CAD build for the part. Positions are in the model's coordinates, mm. Coordinates: 2 decimals unless noted, no trailing zeros. Write each loop counter-clockwise with the first axis right and the second up, starting at its lowest first coordinate (ties: lowest second). Pieces come first, ordered by that corner, then holes. Notation, with made-up numbers: (-31.5, -2) -> (-12.5, -2) arc R18 ccw to (-12.5, 23) -> close; hole circle Ø2 at (66, 7.5). An arc over 180 degrees is marked (long way). Answer as CSV lines item,"result".
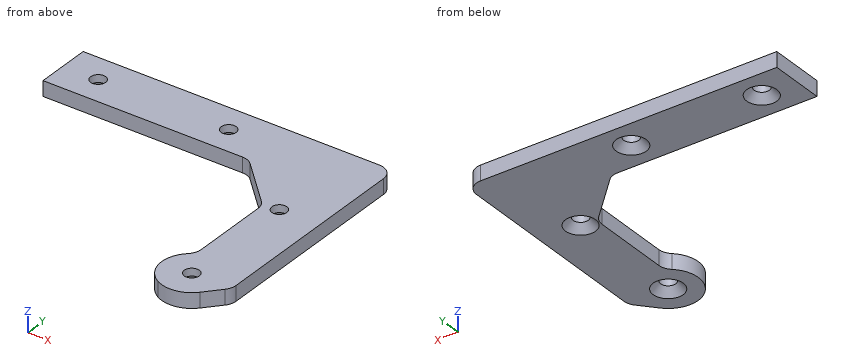
```python
from build123d import *

# Parameters (mm, degrees)
EXTRUDE_598_DEPTH      = 3
SKETCH_656_R           = 1.5
CUT_EXTRUDE_1014_DEPTH = 74.235920149
SKETCH_3_R             = 6
SKETCH_3_R_2           = 1.5
EXTRUDE_1306_DEPTH     = 3
CUT_EXTRUDE_1628_DEPTH = 74.235920149
CHAMFER_3_SIZE         = 10
FILLET_3_R             = 3
CHAMFER_2_SIZE         = 1.5


with BuildPart() as part:
    # Эскиз1 → Extrude 598 (new body)
    with BuildSketch(Plane.XY):
        Polygon((-56.5, 5.5), (-56.5, -5.5), (-5.5, -5.5), (-5.5, -46.5), (5.5, -46.5), (5.5, 5.5), align=None)
    extrude(amount=EXTRUDE_598_DEPTH)

    # Sketch 656 → Cut-Extrude 1014 (cut, through all)
    with BuildSketch(Plane.XY.offset(3)):
        with Locations((-49.5, 0)):
            Circle(SKETCH_656_R)
        with Locations((-23.5, 0)):
            Circle(SKETCH_656_R)
        with Locations((-2.5, -15)):
            Circle(SKETCH_656_R)
        with Locations((-2.5, -39)):
            Circle(SKETCH_656_R)
    extrude(amount=-CUT_EXTRUDE_1014_DEPTH, mode=Mode.SUBTRACT)

    # Эскиз3 → Extrude 1306 (add)
    with BuildSketch(Plane.XY.offset(3)):
        with Locations((-2.5, -39)):
            Circle(SKETCH_3_R)
        with Locations((-2.5, -39)):
            Circle(SKETCH_3_R_2, mode=Mode.SUBTRACT)
    extrude(amount=-EXTRUDE_1306_DEPTH)

    # Эскиз4 → Cut-Extrude 1628 (cut, through all)
    with BuildSketch(Plane.XY.offset(3)):
        with BuildLine():
            Line((-5.5, -46.5), (-5.5, -44.196152423))
            ThreePointArc((-5.5, -44.196152423), (-1.530874267, -44.921215696), (2, -42.968626967))
            Line((2, -42.968626967), (5.5, -39))
            Line((5.5, -39), (5.5, -46.5))
            Line((5.5, -46.5), (-5.5, -46.5))
        make_face()
    extrude(amount=-CUT_EXTRUDE_1628_DEPTH, mode=Mode.SUBTRACT)

    # Фаска3
    chamfer_3_edges = [part.edges().sort_by_distance(p)[0] for p in [
        (-5.5, -5.5, 1.5),
    ]]
    chamfer(chamfer_3_edges, length=CHAMFER_3_SIZE)

    # Скругление3
    fillet_3_edges = [part.edges().sort_by_distance(p)[0] for p in [
        (5.5, 5.5, 1.5),
        (-5.5, -33.803847577, 1.5),
        (5.5, -39, 1.5),
        (-5.5, -15.5, 1.5),
        (-15.5, -5.5, 1.5),
    ]]
    fillet(fillet_3_edges, radius=FILLET_3_R)

    # Фаска2
    chamfer_2_edges = [part.edges().sort_by_distance(p)[0] for p in [
        (-4, -15, 0),
        (-51, 0, 0),
        (-25, 0, 0),
        (-4, -39, 0),
    ]]
    chamfer(chamfer_2_edges, length=CHAMFER_2_SIZE)


solid = part.part
```
Item 1: Saw through at A-A on x = -2.5. Give the cut face in (y, z), and give its area (3 significant figures).
Answer below:
outline,"(-45, 0) -> (-42, 0) -> (-40.5, 1.5) -> (-40.5, 3) -> (-45, 3) -> close; (-37.5, 1.5) -> (-36, 0) -> (-18, 0) -> (-16.5, 1.5) -> (-16.5, 3) -> (-37.5, 3) -> close; (-13.5, 1.5) -> (-12, 0) -> (5.5, 0) -> (5.5, 3) -> (-13.5, 3) -> close"
area,"129 mm2"
Item 2: Saw through at C-C on z = 0.95. Give the cut face in (x, y).
Answer below:
outline,"(-56.5, -5.5) -> (-16.74, -5.5) arc R3 cw to (-14.62, -6.38) -> (-6.38, -14.62) arc R3 cw to (-5.5, -16.74) -> (-5.5, -32.29) arc R3 cw to (-6.5, -34.53) arc R6 ccw (long way) to (2, -42.97) -> (4.75, -39.85) arc R3 ccw to (5.5, -37.87) -> (5.5, 2.5) arc R3 ccw to (2.5, 5.5) -> (-56.5, 5.5) -> close; hole circle Ø4.1 at (-49.5, 0); hole circle Ø4.1 at (-23.5, 0); hole circle Ø4.1 at (-2.5, -39); hole circle Ø4.1 at (-2.5, -15)"
Item 3: Saw through at D-D on x = -23.5. Give the cut face in (y, z), and give its area (4 significant figures).
Answer below:
outline,"(-5.5, 0) -> (-3, 0) -> (-1.5, 1.5) -> (-1.5, 3) -> (-5.5, 3) -> close; (1.5, 1.5) -> (3, 0) -> (5.5, 0) -> (5.5, 3) -> (1.5, 3) -> close"
area,"21.75 mm2"
Item 4: Saw through at B-B on y = 0. Give the cut face in (x, z), and give its area (4 significant figures).
Answer below:
outline,"(-56.5, 0) -> (-52.5, 0) -> (-51, 1.5) -> (-51, 3) -> (-56.5, 3) -> close; (-48, 1.5) -> (-46.5, 0) -> (-26.5, 0) -> (-25, 1.5) -> (-25, 3) -> (-48, 3) -> close; (-22, 1.5) -> (-20.5, 0) -> (5.5, 0) -> (5.5, 3) -> (-22, 3) -> close"
area,"163.5 mm2"
Item 5: Wall check: line 1 (Y direction, x = -2.5, z = 2.45); line 2 (X direction, y = 0.5, z = 0.85); line 3 (Y direction, x = -23.5, z = 2.25). Give the ranges that are in metal, low to high. Write a range as from..to.
Answer below:
line 1,"y = -45..-40.5, -37.5..-16.5, -13.5..5.5"
line 2,"x = -56.5..-51.59, -47.41..-25.59, -21.41..5.5"
line 3,"y = -5.5..-1.5, 1.5..5.5"
Item 6: Flat gauge pins, fed straight in: pin 1 (1 mm diameter, centred on x = -25.5, z = 2.5, fed in from -Y); pin 2 (1.5 mm diameter, centred on y = -28.5, z = 2, fed in from -X); pin 3 (1.5 mm diameter, centred on x = -12, z = 1.5, fed in from -Y). Where does each tip first touch, or does it go through?
Answer below:
pin 1,"stops at y = -5.5"
pin 2,"stops at x = -5.5"
pin 3,"stops at y = -9.75"
